Check sheet for the modelled part. Datum: model origin and axes. Units: mm. Face numbers are marked on the shaded views. A direction names the side the tool comes from. Coordinates: 2 decimals unless noted, no trailing zeros. Order: outer loops, then holes, each group sorted by start corner. A loop starts at its lowest first (then second) coordinate and runs counter-clockwise, first axis right, second up.
1. Draft check along Y on the marked faces 1, 2, 3 and 4. Enter one of: released by +Y, released by -Y, zero draft, split by the parting line, or undercut.
2. Cross-section at B-B (z = -9.5). Enter the section's corners in (x, y), then the cut area to 3 significant figures.
3. Cross-section at A-A (y = 715). Enter the section's corners in (x, z), then the cut area to 3 significant figures.
4. Cross-section at D-D (z = 194.5). Enter the section's corners in (x, y).
5. Thickness scan on line 1 (Y direction, x = 315.5, z = -65.5); line 2 (X direction, y = -912, z = -38.5); line 3 (Z direction, x = -501, y = 610). Record the ranges inside material, lowest first.
6. Set-up check for the marked faces 5 and 6: record each of +Z, -Z, +X, -X, +Y, -Y from which the full face is reachable in a straight line by a thin tool's end or side.
7. Gauge pin test, flat ends, axial feed: pin 1 Ø9 at (x, y) = (316.5, 1065.5) entering from +Z; pin 2 Ø15 at (x, y) = (331.5, 1060) entering from -Z. Record the tip position at first contact, or that the pin passes through.
8. Cross-section at C-C (x = 100.5). Enter the section's corners in (y, z).
```python
from build123d import *

# Parameters (mm, degrees)
ESBO_O1_W                     = 1200
ESBO_O1_H                     = 2300
ESBO_O1_W_2                   = 1000
ESBO_O1_H_2                   = 2100
EXTRUS_O_FINA1_DEPTH          = 100
RESSALTO_EXTRUS_O1_DEPTH      = 200
RESSALTO_EXTRUS_O1_DEPTH_BACK = 400
ESBO_O2_W                     = 1200
ESBO_O2_H                     = 100
ESBO_O3_W                     = 70
ESBO_O3_H                     = 17
CORTE_EXTRUS_O1_DEPTH         = 30


with BuildPart() as part:
    # Esboço1 → Extrusão-Fina1 (new, symmetric)
    with BuildSketch(Plane.XY):
        Rectangle(ESBO_O1_W, ESBO_O1_H)
        Rectangle(ESBO_O1_W_2, ESBO_O1_H_2, mode=Mode.SUBTRACT)
    extrude(amount=EXTRUS_O_FINA1_DEPTH, both=True)

    # Esboço2 → Ressalto-extrusão1 (add, two sides: drawn at the far end of the back side and taken through both)
    with BuildSketch(Plane.XY.offset(100).offset(-RESSALTO_EXTRUS_O1_DEPTH_BACK)):
        with Locations((0, -1100)):
            Rectangle(ESBO_O2_W, ESBO_O2_H)
    extrude(amount=RESSALTO_EXTRUS_O1_DEPTH + RESSALTO_EXTRUS_O1_DEPTH_BACK)

    # Esboço3 → Corte-extrusão1 (cut)
    with BuildSketch(Plane.XZ.offset(-1050)):
        with Locations((320, 74)):
            Rectangle(ESBO_O3_W, ESBO_O3_H)
    extrude(amount=-CORTE_EXTRUS_O1_DEPTH, mode=Mode.SUBTRACT)


solid = part.part
```
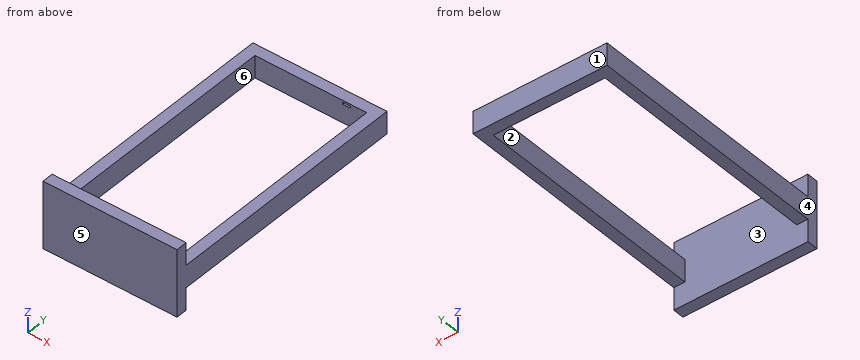
Data:
1. face 1: released by +Y
1. face 2: undercut
1. face 3: undercut
1. face 4: zero draft
2. outline: (-600, -1150) - (600, -1150) - (600, 1150) - (-600, 1150) - close; hole (-500, -1050) - (500, -1050) - (500, 1050) - (-500, 1050) - close
2. area: 660,000 mm2
3. outline: (-600, -100) - (-500, -100) - (-500, 100) - (-600, 100) - close; (500, -100) - (600, -100) - (600, 100) - (500, 100) - close
3. area: 40,000 mm2
4. outline: (-600, -1150) - (600, -1150) - (600, -1050) - (-600, -1050) - close
5. line 1: y = -1150 to -1050, 1050 to 1150
5. line 2: x = -600 to -500, 500 to 600
5. line 3: z = -100 to 100
6. face 5: +Z, -Z, +X, -X, -Y
6. face 6: +Z, -Z
7. pin 1: stops at z = 100
7. pin 2: stops at z = -100
8. outline: (-1150, -300) - (-1050, -300) - (-1050, 300) - (-1150, 300) - close; (1050, -100) - (1150, -100) - (1150, 100) - (1050, 100) - close
